Here's the drawing with two shaded views (mm, measured from the low corner). I have some questions. A direction names the side the tool comes from. Round coordinates to 2 decimals unless told otherwise and drop trailing zeros. Order: outer loops, then holes, each group sorted by start corner. A loop starts at its lowest first (then second) coordinate and runs counter-clockwise, first axis right, second up.
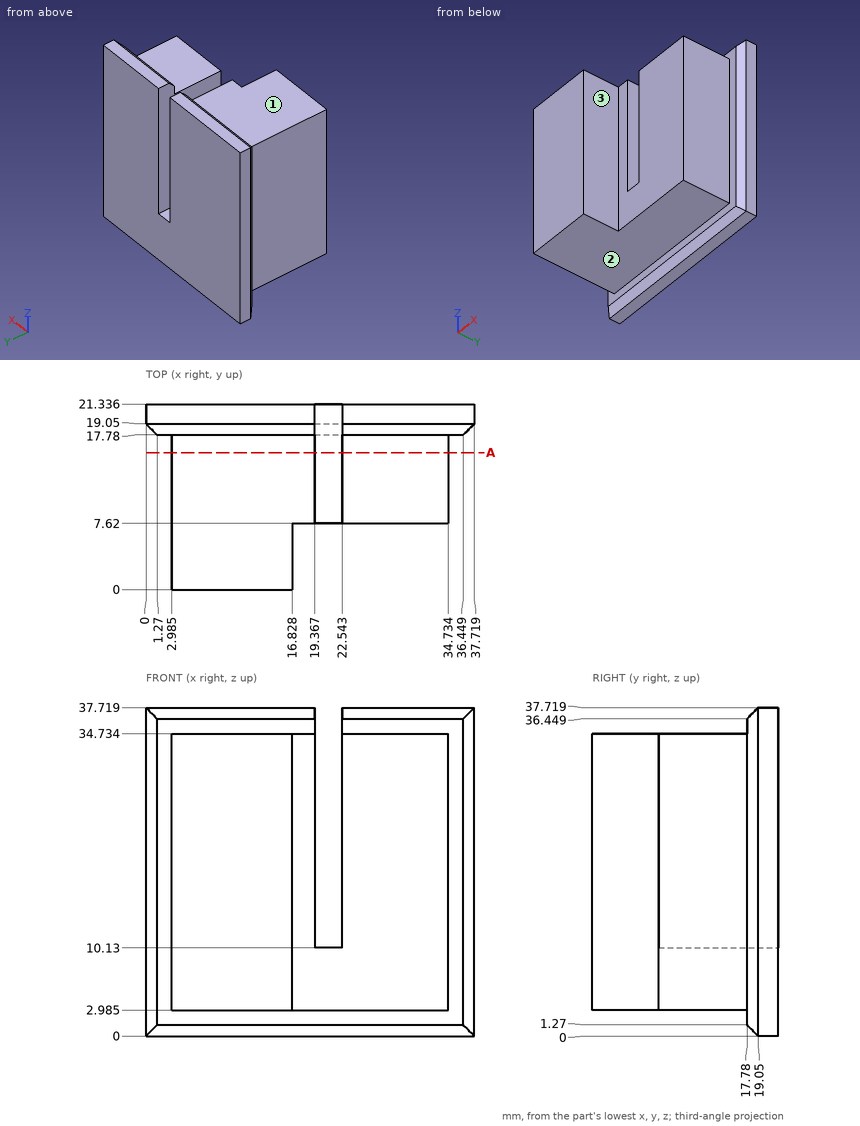
Q1. I need wall thicknesses on L1, parallel to X at y = 11.75, z = 21 (1 decimal); L2, parallel to Z at x = 7, y = 9.5 (1 decimal); L3, parallel to X at y = 1, z = 12.5 (1 decimal). Which ranges of each line are inside material? Lowest first, please.
Q2. For P1, Ø8, axis at x = 11.5, y = 6, coming from the +Z side (1 decimal); P2, Ø11, axis at y = 12, z = 26, coming from the +X side (1 decimal); P3, Ø6, axis at y = 3, z = 10, coming from the +X side; P4, Ø1.5, axis at x = 20.5, z = 30.5, coming from the +Y side, each with a flat end and sliding along its axis, tell me the tip position at first contact or that it passes through.
Q3. For the marked faces 1, 2 and 3, which set-ups out of +Z, -Z, +X, -X, +Y, -Y let a thin tool reach every point of the face, with its end or its side?
Q4. Imagine slicing it at A-A, the plane y = 15.75. Please give me the cut outline in (x, z) (1 decimal).
Filled in:
1. L1: x = 3 to 19.4, 22.5 to 34.7
1. L2: z = 3 to 34.7
1. L3: x = 3 to 16.8
2. P1: stops at z = 34.7
2. P2: stops at x = 34.7
2. P3: stops at x = 16.83
2. P4: passes through
3. face 1: +Z, +X, -X, -Y
3. face 2: -Z, +X, -X, -Y
3. face 3: +Z, -Z, +X, -Y
4. outline: (3, 3) - (34.7, 3) - (34.7, 34.7) - (22.5, 34.7) - (22.5, 10.1) - (19.4, 10.1) - (19.4, 34.7) - (3, 34.7) - close
